Geometry check sheet. Reference: drawing and pictorial views, mm from the part's lowest x, y, z. A direction names the side the tool comes from. Round coordinates to 2 decimals unless told otherwise and drop trailing zeros. Write each loop counter-clockwise with the first axis right and the second up, starting at its lowest first coordinate (ties: lowest second). Pieces come first, ordered by that corner, then holes. Notation, with made-up numbers: (64.5, 72.25) - (109.5, 72.25) arc R24 cw to (109.5, 106.25) - close; hole circle Ø9 at (25, 57). An arc over 180 degrees is marked (long way). Use one line per item in the form item = value. Start each with the question number.
1) Draft check along Y on the marked faces 1, 2 and 3. Enter one of: +Y half, -Y half, draft (parallel to the pull), parting line (faces both ways), or undercut.
2) Section check B-B (z = 12.25). Record the boundary of the cut face in (x, y), then the cut area to 3 significant figures.
3) Section check A-A (x = 161.5). Record the boundary of the cut face in (y, z), then the cut area to 3 significant figures.
4) Scan lines: probe 1 along Y at (x, z) = (171, 14.5); probe 2 along X at (y, z) = (309, 8.25). Record each from-to range of solid material in increasing order.
5) Section check C-C (y = 164). Record the boundary of the cut face in (x, z).
6) Gauge pin test, flat ends, axial feed: P1, Ø12.5, axis at y = 124, z = 6.5, coming from the +X side; P2, Ø5, axis at y = 58.5, z = 11.5, coming from the -X side; P3, Ø12.5, axis at y = 131.5, z = 9, coming from the -X side; P4, Ø12.5, axis at x = 167, z = 16, coming from the -Y side. Record the tip position at first contact, or that the pin passes through.
7) Set-up check for the marked faces 4, 5, 6, 7 and 8: record each of +Z, -Z, +X, -X, +Y, -Y from which the full face is reachable in a straight line by a thin tool's end or side.
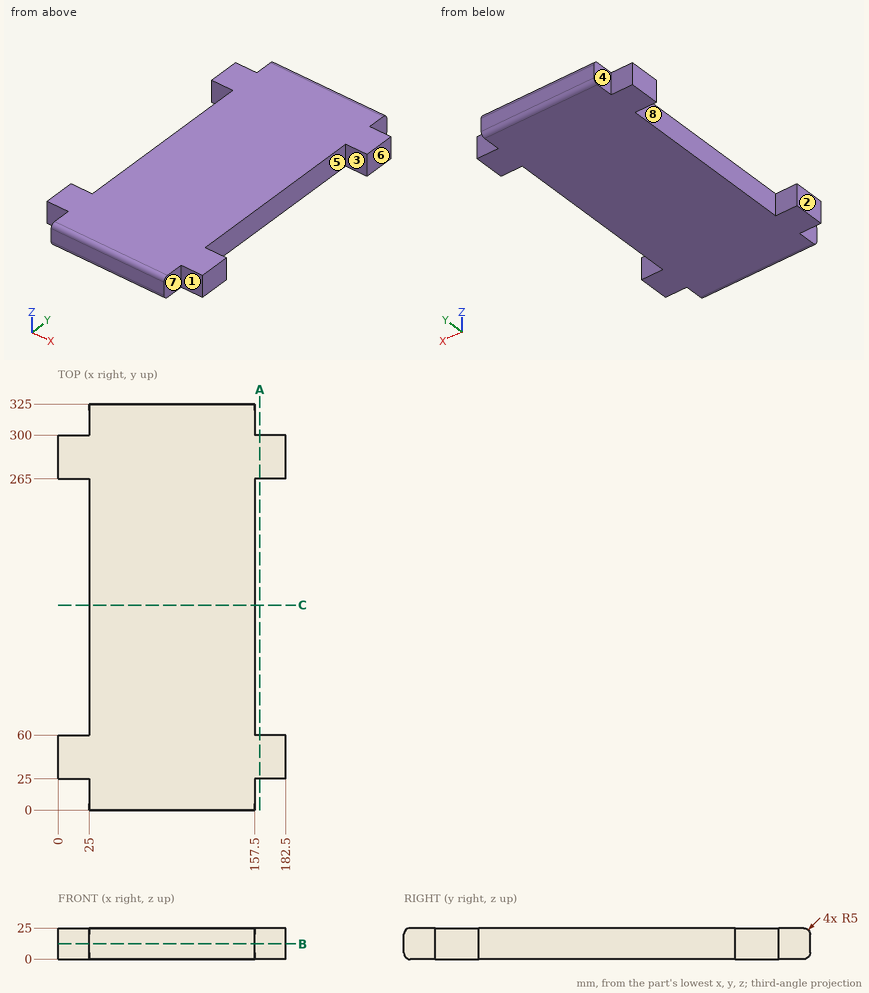
Results are:
q1.face_1 = -Y half
q1.face_2 = draft
q1.face_3 = undercut
q2.outline = (0, 25) - (25, 25) - (25, 0) - (157.5, 0) - (157.5, 25) - (182.5, 25) - (182.5, 60) - (157.5, 60) - (157.5, 265) - (182.5, 265) - (182.5, 300) - (157.5, 300) - (157.5, 325) - (25, 325) - (25, 300) - (0, 300) - (0, 265) - (25, 265) - (25, 60) - (0, 60) - close
q2.area = 46,600 mm²
q3.outline = (25, 0) - (60, 0) - (60, 25) - (25, 25) - close; (265, 0) - (300, 0) - (300, 25) - (265, 25) - close
q3.area = 1,750 mm²
q4.probe_1 = 25 to 60, 265 to 300
q4.probe_2 = 25 to 157.5
q5.outline = (25, 0) - (157.5, 0) - (157.5, 25) - (25, 25) - close
q6.P1 = 157.5
q6.P2 = 0
q6.P3 = 25
q6.P4 = 25
q7.face_4 = +Z, -Z, -X, +Y
q7.face_5 = +Z, -Z, +X
q7.face_6 = +Z, -Z, +X, +Y, -Y
q7.face_7 = +Z, -Z, +X, -Y
q7.face_8 = +Z, -Z, -X
